```python
from build123d import *

# Parameters (mm, degrees)
BOSS_EXTRUDE1_DEPTH       = 5.5
SKETCH3_OUTSIDE_W         = 37.596
SKETCH3_OUTSIDE_H         = 36.12
SKETCH3_OUTSIDE_R         = 8
CUT_EXTRUDE1_DEPTH        = 5.5
CUT_EXTRUDE1_DRAFT        = -45
F_4_0MM_DOWEL_HOLE1_D     = 4
F_4_0MM_DOWEL_HOLE1_DEPTH = 16
F_4_0MM_DOWEL_HOLE1_TIP   = 1.201721238
CUT_EXTRUDE2_REACH        = 28.904
SKETCH6_R                 = 2


with BuildPart() as part:
    # Sketch1 → Revolve1 (revolve)
    with BuildSketch(Plane.XY, mode=Mode.PRIVATE) as revolve1_sk:
        with BuildLine():
            Line((0, 0), (-5, 0))
            Line((-5, 0), (-6, 1))
            Line((-6, 1), (-6, 8.5))
            ThreePointArc((-6, 8.5), (-5.25, 9.25), (-6, 10))
            Line((-6, 10), (-8.5, 10))
            Line((-8.5, 10), (-8.5, 12))
            Line((-8.5, 12), (0, 12))
            Line((0, 12), (0, 0))
        make_face()
    revolve(revolve1_sk.sketch.rotate(Axis((0, 12, 0), (0, -1, 0)), 270), axis=Axis((0, 12, 0), (0, -1, 0)))

    # Sketch2 → Boss-Extrude1 (add)
    with BuildSketch(Plane(origin=(0, 12, 0), x_dir=(1, 0, 0), z_dir=(0, 1, 0))):
        Polygon((-4.618802154, 8), (-9.237604307, 0), (-4.618802154, -8), (4.618802154, -8), (9.237604307, 0), (4.618802154, 8), align=None)
    extrude(amount=BOSS_EXTRUDE1_DEPTH)


with BuildPart() as cut_extrude1_tool:
    # Sketch3 outside → Cut-Extrude1 (with draft: the straight prism first)
    with BuildSketch(Plane(origin=(0, 17.5, 0), x_dir=(1, 0, 0), z_dir=(0, 1, 0))):
        Rectangle(SKETCH3_OUTSIDE_W, SKETCH3_OUTSIDE_H)
        Circle(SKETCH3_OUTSIDE_R, mode=Mode.SUBTRACT)
    extrude(amount=-CUT_EXTRUDE1_DEPTH)
    # Cut-Extrude1: the draft: its side faces are tilted about the plane it starts from
    cut_extrude1_sides = [cut_extrude1_tool.faces().sort_by_distance(p)[0] for p in [
        (0, 14.75, 18.06),
        (18.798, 14.75, 0),
        (0, 14.75, -18.06),
        (-18.798, 14.75, 0),
        (-8, 14.75, 0),
    ]]
    draft(cut_extrude1_sides, Plane(origin=(0, 17.5, 0), x_dir=(1, 0, 0), z_dir=(0, 1, 0)), CUT_EXTRUDE1_DRAFT)


with BuildPart() as part_1:
    add(part.part)

    # Cut-Extrude1: cut by cut_extrude1_tool
    add(cut_extrude1_tool.part, mode=Mode.SUBTRACT)

    # Ø4.0mm Dowel Hole1
    with Locations(Plane(origin=(0, 0, 0), x_dir=(-1, 0, 0), z_dir=(0, -1, 0))):
        with Locations((0, 0)):
            Hole(F_4_0MM_DOWEL_HOLE1_D / 2, depth=F_4_0MM_DOWEL_HOLE1_DEPTH)
            with Locations((0, 0, -(F_4_0MM_DOWEL_HOLE1_DEPTH + F_4_0MM_DOWEL_HOLE1_TIP / 2))):  # 118° drill point
                Cone(0, F_4_0MM_DOWEL_HOLE1_D / 2, F_4_0MM_DOWEL_HOLE1_TIP, mode=Mode.SUBTRACT)

    # Sketch6 → Cut-Extrude2 (cut, up to next)
    with BuildSketch(Plane(origin=(6.92820323, 0, 4), x_dir=(0.5, 0, -0.8660254037844386), z_dir=(0.8660254037844387, 0, 0.5000000000000001)), mode=Mode.PRIVATE) as cut_extrude2_sk1:
        with Locations((0, 14.75)):
            Circle(SKETCH6_R)
    cut_extrude2_tool1 = extrude(cut_extrude2_sk1.sketch, amount=-CUT_EXTRUDE2_REACH, mode=Mode.PRIVATE) & part_1.part
    add(cut_extrude2_tool1.solids().sort_by_distance((6.928203, 14.75, 4))[0], mode=Mode.SUBTRACT)


solid = part_1.part
```
Input: part model. Units: mm. Frame: model coordinates. A direction names the side the tool comes from. Give positions to 0.01 mm unless a question says otherwise; leave off trailing zeros. Order: outer loops, then holes, each group sorted by start corner. A loop starts at its lowest first (then second) coordinate and runs counter-clockwise, first axis right, second up. Notation, with made-up numbers: M 42,45.5 L 87,45.5 A27 ccw 87,79.5 Z; hole C -35.75,5 d6. An arc over 180 degrees is marked long. Return JSON: item names as keys, results as strings.
Item 1: First-contact query: P1, Ø8, axis at x = -3, y = 9, coming from the +Z side; P2, Ø2, axis at y = 4.5, z = 1.5, coming from the -X side; P3, Ø5, axis at y = 2.5, z = -6.5, coming from the +X side; P4, Ø4, axis at x = 6.5, z = 4, coming from the -Y side. Flat tips, straight axial feed; report the tip coordinate or a pass-through.
Solutions:
{"P1": "z = 8.5", "P2": "x = -5.98", "P3": "x = 4.47", "P4": "y = 0.63"}
Item 2: Ray query, probe 1 along Y at (x, z) = (7.5, 3.5); probe 2 along Y at (x, z) = (2.25, -7.25); probe 3 along Z at (x, y) = (-6, 10.5). Return the intervals inside material, ascending.
Solutions:
{"probe 1": "10 to 12", "probe 2": "10 to 17.5", "probe 3": "-6.02 to 6.02"}
Item 3: Cut plane A-A (y = 6.75). Return loops of the section in (x, z), then the cut area to 3 significant figures.
Solutions:
{"outline": "C 0,0 d12; hole C 0,0 d4", "area": "101 mm^2"}
Item 4: Access query for faces 1 (the flat face through (6.961, 14.711, -3.944)), 2 (the flat face through (-7.1, 12, -4.2)), 3 (the flat face through (-4.4, 12, -7.6)). Directions: +Z, -Z, +X, -X, +Y, -Y. A direction counts if a zero-diameter tool reaches every point of the face in a straight line with its end or side. Return the directions, or none.
Solutions:
{"face 1": "-Z, +X, +Y", "face 2": "-Z, -X, +Y", "face 3": "-Z, -X, -Y"}
